Verification items for the finished model (mm, model axes). A direction names the side the tool comes from. Coordinates: 2 decimals unless noted, no trailing zeros. Loops run counter-clockwise (first coordinate to the right, second up) from the corner with the lowest first, then second, coordinate; pieces in that order, holes last. Notation, with made-up numbers: (-31.75, 45) -> (16.25, 45) arc R20 cw to (16.25, 63) -> close; hole circle Ø10 at (11, 24.5). An arc over 180 degrees is marked (long way). Answer as a JSON object with one key per item and string values. Group by question number.
Q1. Release check for a two-part mould opening along X. For faces 3 (the flat face through (-100, -135, -88)), 4 (the conical face through (26.67, -29.96, 8.4)), 5 (the conical face through (37.31, -25.865, -15.47)) record: released by +X, released by -X, zero draft, split by the parting line, or undercut.
Q2. Cross-section at B-B on y = -27.5. Record the boundary of the cut face in (x, z) (3 decimals), and give its area (3 significant figures).
Q3. Scan lines: L1, parallel to X at y = -7, z = 0 (3 decimals); L2, parallel to Z at x = -23, y = -102; L3, parallel to X at y = -4.5, z = 0 (3 decimals). Record each from-to range of solid material in increasing order.
Q4. Gauge pin test, flat ends, axial feed: pin 1 Ø4 at (x, z) = (-66, -72.5) entering from +Y; pin 2 Ø6 at (x, y) = (76, -104.5) entering from +Z; pin 3 Ø5 at (x, y) = (-2, 3) entering from -Z. Record the tip position at first contact, or that the pin passes through.
Q5. Set-up check for faces 1 (the flat face through (0, 5, -8.001)), 2 (the flat face through (0, 10, 9)): record each of +Z, -Z, +X, -X, +Y, -Y from which the full face is reachable in a straight line by a thin tool's end or side.
Q6. Cross-section at A-A on y = -95. Record the boundary of the cut face in (x, z) (3 decimals), and give its area (3 significant figures).
```python
from build123d import *

# Parameters (mm, degrees)
SKETCH1_R                                   = 14.525
KEYED_PORTION_ADAPTER_DEPTH                 = 10
STOPPER_START                               = 10
SKETCH2_R                                   = 14.525
SKETCH2_R_2                                 = 8.001087489
STOPPER_ON_THREADED_PORTION_OF_PISTON_DEPTH = 10
PISTON_HOLDER_TO_CONICAL_BASE_ADAPTER_R     = 10


with BuildPart() as part:
    # Sketch1 → Keyed portion adapter (new body)
    with BuildSketch(Plane(origin=(0, 0, 0), x_dir=(1, 0, 0), z_dir=(0, 1, 0))):
        with Locations(Location((0, 0, 0), (0, 0, 270))):
            Circle(SKETCH1_R)
        with BuildLine():
            Line((-5.168, 8.001087489), (5.168, 8.001087489))
            ThreePointArc((5.168, 8.001087489), (9.525, 0), (5.168, -8.001087489))
            Line((5.168, -8.001087489), (-5.168, -8.001087489))
            ThreePointArc((-5.168, -8.001087489), (-9.525, 0), (-5.168, 8.001087489))
        make_face(mode=Mode.SUBTRACT)
    extrude(amount=KEYED_PORTION_ADAPTER_DEPTH)

    # Sketch2 → Stopper (on threaded portion of piston) (add)
    with BuildSketch(Plane.XZ.offset(STOPPER_START)):
        with Locations(Location((0, 0, 0), (0, 0, 270))):
            Circle(SKETCH2_R)
        with Locations(Location((0, 0, 0), (0, 0, 270))):
            Circle(SKETCH2_R_2, mode=Mode.SUBTRACT)
    extrude(amount=-STOPPER_ON_THREADED_PORTION_OF_PISTON_DEPTH)

    # Sketch3 → Conical base (revolve)
    with BuildSketch(Plane.XY):
        Polygon((8.001087489, -10), (8.001087489, 0), (14.525, 0), (149.525, -135), (133.001087489, -135), align=None)
    revolve(axis=Axis((0, 0, 0), (0, -1, 0)))

    # Piston holder to conical base adapter
    piston_holder_to_conical_base_adapter_edges = [part.edges().sort_by_distance(p)[0] for p in [
        (-10.270725997, 0, -10.270725997),
    ]]
    fillet(piston_holder_to_conical_base_adapter_edges, radius=PISTON_HOLDER_TO_CONICAL_BASE_ADAPTER_R)


solid = part.part
```
Computed values:
{
 "1": {"face 3": "zero draft", "face 4": "undercut", "face 5": "split by the parting line"},
 "2": {"outline": "circle Ø84.05 at (0, 0); hole circle Ø51.002 at (0, 0)", "area": "3,510 mm²"},
 "3": {"L1": "x = -21.525 to -8.001, 8.001 to 21.525", "L2": "z = -114.23 to -97.32, 97.32 to 114.23", "L3": "x = -19.025 to -8.001, 8.001 to 19.025"},
 "4": {"pin 1": "stops at y = -81.52", "pin 2": "stops at z = 96.14", "pin 3": "stops at z = -15.12"},
 "5": {"face 1": "+Y", "face 2": "+Z, -Z, +X, -X, +Y"},
 "6": {"outline": "circle Ø219.05 at (0, 0); hole circle Ø186.002 at (0, 0)", "area": "10,500 mm²"}
}
